Here's how the part is built. I have some questions about the finished solid (model axes, mm). A direction names the side the tool comes from. Round coordinates to 2 decimals unless told otherwise and drop trailing zeros. Loops run counter-clockwise (first coordinate to the right, second up) from the corner with the lowest first, then second, coordinate; pieces in that order, holes last. Notation, with made-up numbers: M 63.25,65 L 76.25,65 A10 ccw 76.25,75 Z; hole C -21.5,4.5 d11. An arc over 180 degrees is marked long. Use a Markdown table: item, result.
```python
from build123d import *

# Parameters (mm, degrees)
CROQUIS1_W                = 50
CROQUIS1_H                = 50
SALIENTE_EXTRUIR1_DEPTH   = 625
SALIENTE_EXTRUIR1_2_DEPTH = 625
SALIENTE_EXTRUIR1_3_DEPTH = 625
SALIENTE_EXTRUIR1_4_DEPTH = 625
CROQUIS2_W                = 90
CROQUIS2_H                = 90
SALIENTE_EXTRUIR2_DEPTH   = 50
CROQUIS4_W                = 50
CROQUIS4_H                = 50
SALIENTE_EXTRUIR3_DEPTH   = 853
SALIENTE_EXTRUIR4_DEPTH   = 50


with BuildPart() as part:
    # Croquis1 → Saliente-Extruir1 (new body)
    with BuildSketch(Plane(origin=(0, 0, 0), x_dir=(1, 0, 0), z_dir=(0, 1, 0))):
        with Locations((-237.132034356, 237.132034356)):
            Rectangle(CROQUIS1_W, CROQUIS1_H)
    extrude(amount=-SALIENTE_EXTRUIR1_DEPTH)



with BuildPart() as body_2:
    # Croquis1 → Saliente-Extruir1 2 (new body)
    with BuildSketch(Plane(origin=(0, 0, 0), x_dir=(1, 0, 0), z_dir=(0, 1, 0))):
        with Locations((237.132034356, 237.132034356)):
            Rectangle(CROQUIS1_W, CROQUIS1_H)
    extrude(amount=-SALIENTE_EXTRUIR1_2_DEPTH)


with BuildPart() as body_3:
    # Croquis1 → Saliente-Extruir1 3 (new body)
    with BuildSketch(Plane(origin=(0, 0, 0), x_dir=(1, 0, 0), z_dir=(0, 1, 0))):
        with Locations((-237.132034356, -237.132034356)):
            Rectangle(CROQUIS1_W, CROQUIS1_H)
    extrude(amount=-SALIENTE_EXTRUIR1_3_DEPTH)


with BuildPart() as body_4:
    # Croquis1 → Saliente-Extruir1 4 (new body)
    with BuildSketch(Plane(origin=(0, 0, 0), x_dir=(1, 0, 0), z_dir=(0, 1, 0))):
        with Locations((237.132034356, -237.132034356)):
            Rectangle(CROQUIS1_W, CROQUIS1_H)
    extrude(amount=-SALIENTE_EXTRUIR1_4_DEPTH)


with BuildPart() as part_1:
    add(part.part)

    add(body_2.part)  # Saliente-Extruir2 merges body 2

    add(body_3.part)  # Saliente-Extruir2 merges body 3

    add(body_4.part)  # Saliente-Extruir2 merges body 4
    # Croquis2 → Saliente-Extruir2 (add)
    with BuildSketch(Plane.XZ.offset(625)):
        with Locations((-237.132034356, 237.132034356)):
            Rectangle(CROQUIS2_W, CROQUIS2_H)
        with Locations((237.132034356, 237.132034356)):
            Rectangle(CROQUIS2_W, CROQUIS2_H)
        with Locations((237.132034356, -237.132034356)):
            Rectangle(CROQUIS2_W, CROQUIS2_H)
        with Locations((-237.132034356, -237.132034356)):
            Rectangle(CROQUIS2_W, CROQUIS2_H)
    extrude(amount=SALIENTE_EXTRUIR2_DEPTH)

    # Croquis4 → Saliente-Extruir3 (add)
    with BuildSketch(Plane.XZ.offset(675)):
        with Locations((-237.132034356, 237.132034356)):
            Rectangle(CROQUIS4_W, CROQUIS4_H)
        with Locations((-237.132034356, -237.132034356)):
            Rectangle(CROQUIS4_W, CROQUIS4_H)
        with Locations((237.132034356, 237.132034356)):
            Rectangle(CROQUIS4_W, CROQUIS4_H)
        with Locations((237.132034356, -237.132034356)):
            Rectangle(CROQUIS4_W, CROQUIS4_H)
    extrude(amount=SALIENTE_EXTRUIR3_DEPTH)

    # Croquis6 → Saliente-Extruir4 (add)
    with BuildSketch(Plane(origin=(0, -800, 0), x_dir=(1, 0, 0), z_dir=(0, 1, 0))):
        Polygon((-262.132034356, 262.132034356), (262.132034356, 262.132034356), (262.132034356, -262.132034356), (212.132034356, -262.132034356), (212.132034356, -212.132034356), (212.132034356, 212.132034356), (-212.132034356, 212.132034356), (-212.132034356, -212.132034356), (-212.132034356, -262.132034356), (-262.132034356, -262.132034356), align=None)
    extrude(amount=-SALIENTE_EXTRUIR4_DEPTH)


solid = part_1.part
```
Q1. Will these pins go through, and if not, where does the flat tip stop? P1, Ø15, axis at y = -405.5, z = -245.5, coming from the +X side; P2, Ø25, axis at y = -189, z = -249, coming from the -X side; P3, Ø15, axis at x = -238, y = -425, coming from the -Z side.
Return value:
| item | result |
|---|---|
| P1 | stops at x = 262.13 |
| P2 | stops at x = -262.13 |
| P3 | stops at z = -262.13 |
Q2. Imagine slicing it at D-D, the plane x = -63. Please give me the cut outline in (y, z).
Return value:
| item | result |
|---|---|
| outline | M -850,-262.13 L -800,-262.13 L -800,-212.13 L -850,-212.13 Z |
Q3. Imagine slicing it at A-A, the plane z = -134.5. Please give me the cut outline in (x, y), then the cut area to 3 significant figures.
Return value:
| item | result |
|---|---|
| outline | M -262.13,-850 L -212.13,-850 L -212.13,-800 L -262.13,-800 Z; M 212.13,-850 L 262.13,-850 L 262.13,-800 L 212.13,-800 Z |
| area | 5,000 mm^2 |
Q4. Imagine slicing it at C-C, the plane y = -96. Please give me the cut outline in (x, z).
Return value:
| item | result |
|---|---|
| outline | M -262.13,-262.13 L -212.13,-262.13 L -212.13,-212.13 L -262.13,-212.13 Z; M -262.13,212.13 L -212.13,212.13 L -212.13,262.13 L -262.13,262.13 Z; M 212.13,-262.13 L 262.13,-262.13 L 262.13,-212.13 L 212.13,-212.13 Z; M 212.13,212.13 L 262.13,212.13 L 262.13,262.13 L 212.13,262.13 Z |
Q5. For faces 4 (the flat face through (-237, -1096, 262.132)), 5 (the flat face through (-212.132, -308, -237)), 6 (the flat face through (237, -650, 192.132)), 7 (the flat face through (-237, -308, -262.132)), 8 (the flat face through (-212.132, -1184, -237)), which set-ups out of +Z, -Z, +X, -X, +Y, -Y let a thin tool reach every point of the face, with its end or its side?
Return value:
| item | result |
|---|---|
| face 4 | +Z, +X, -X, -Y |
| face 5 | +Z, -Z, +Y |
| face 6 | +X, -X, +Y |
| face 7 | -Z, +X, -X, +Y |
| face 8 | +Z, -Z, -Y |
Q6. I need wall thicknesses on line 1 (Z direction, x = -227.5, y = -878.5); line 2 (Z direction, x = -254.5, y = -657.5). Which ranges of each line are inside material? Lowest first, please. Write a range as from..to.
Return value:
| item | result |
|---|---|
| line 1 | z = -262.13..-212.13, 212.13..262.13 |
| line 2 | z = -282.13..-192.13, 192.13..282.13 |
Q7. Imagine slicing it at B-B, the plane y = -660. Please give me the cut outline in (x, z), then the cut area to 3 significant figures.
Return value:
| item | result |
|---|---|
| outline | M -282.13,-282.13 L -192.13,-282.13 L -192.13,-192.13 L -282.13,-192.13 Z; M -282.13,192.13 L -192.13,192.13 L -192.13,282.13 L -282.13,282.13 Z; M 192.13,-282.13 L 282.13,-282.13 L 282.13,-192.13 L 192.13,-192.13 Z; M 192.13,192.13 L 282.13,192.13 L 282.13,282.13 L 192.13,282.13 Z |
| area | 32,400 mm^2 |
Q8. We'd pull the mould along Z, two halves only. Please class faces 1 (the flat face through (237, -308, -262.132)), 2 (the flat face through (237, -1184, -212.132)), 3 (the flat face through (212.132, -308, -237)): pulls with the +Z half, pulls with the -Z half, needs draft (parallel to the pull), parting line crosses it, or undercut.
Return value:
| item | result |
|---|---|
| face 1 | pulls with the -Z half |
| face 2 | undercut |
| face 3 | needs draft |
